from build123d import *

# Parameters (mm, degrees)
F1_DEPTH = 12.7
F2_R     = 2.032
F3_DEPTH = 101.601
F4_R     = 2.032
F5_DEPTH = 101.601
F6_R     = 4.953
F7_DEPTH = 63.246
F9_START = 18.542
F8_R     = 4.953
F9_DEPTH = 49.53


with BuildPart() as f1:
    # F0 (on Top) → F1 (new body)
    with BuildSketch(Plane.XY):
        with BuildLine():
            Line((101.6, 99.2), (101.6, 101.6))
            Line((101.6, 101.6), (0, 101.6))
            Line((0, 101.6), (0, 0))
            Line((0, 0), (2.4, 0))
            ThreePointArc((2.4, 0), (31.4550073063, 70.1449926937), (101.6, 99.2))
        make_face()
        with BuildLine():
            Line((2.4, 99.2), (79.6473236256, 99.2))
            ThreePointArc((79.6473236256, 99.2), (29.7579510314, 71.8420489686), (2.4, 21.9526763744))
            Line((2.4, 21.9526763744), (2.4, 99.2))
        make_face(mode=Mode.SUBTRACT)
    extrude(amount=F1_DEPTH)

    # F2 (on Right) → F3 (cut, through all)
    with BuildSketch(Plane.YZ):
        with Locations((19.05, 6.35)):
            Circle(F2_R)
        with BuildLine():
            ThreePointArc((88.532, 6.35), (86.5, 8.382), (84.468, 6.35))
            ThreePointArc((84.468, 6.35), (86.5, 4.318), (88.532, 6.35))
        make_face()
    extrude(amount=F3_DEPTH, mode=Mode.SUBTRACT)

    # F4 (on Front) → F5 (cut, through all)
    with BuildSketch(Plane.XZ):
        with Locations((15.1, 6.35)):
            Circle(F4_R)
        with Locations((88.9, 6.35)):
            Circle(F4_R)
    extrude(amount=-F5_DEPTH, mode=Mode.SUBTRACT)

    # F6 (on Front) → F7 (cut)
    with BuildSketch(Plane.XZ):
        with Locations((15.1, 6.35)):
            Circle(F6_R)
    extrude(amount=-F7_DEPTH, mode=Mode.SUBTRACT)

    # F8 (on Right) → F9 (cut)
    with BuildSketch(Plane.YZ.offset(F9_START)):
        with Locations((86.5, 6.35)):
            Circle(F8_R)
    extrude(amount=F9_DEPTH, mode=Mode.SUBTRACT)


solid = f1.part
Read the model definition and answer for the solid it produces. Units are mm, in the model's axes. A direction names the side the tool comes from. Round coordinates to 2 decimals unless told otherwise and drop trailing zeros. Order: outer loops, then holes, each group sorted by start corner. A loop starts at its lowest first (then second) coordinate and runs counter-clockwise, first axis right, second up.
1) Flat-ended cylindrical pins translate along their axes: pin 1 (6 mm diameter, centred on y = 42.5, z = 9, fed in from +X); pin 2 (5.5 mm diameter, centred on y = 19.05, z = 6.35, fed in from +X) (3 decimals); pin 3 (1 mm diameter, centred on y = 86.5, z = 3, fed in from +X). Find the tip coordinate at first contact, or state that the pin passes through.
2) The part is cut by section D-D on z = 6.35. Give the number of separate pieces and of enclosed holes in the cut face, plus the area to 3 significant figures.
3) The part is cut by section C-C on y = 86.5. Write down the section's boundary in (x, z).
4) Straight lines are drawn through the part: L1, parallel to Y at x = 1.25, z = 6.35; L2, parallel to Z at x = 3.55, y = 19.05; L3, parallel to Y at x = 17, z = 10.25. For each, find the intervals that lie inside material, in ascending order.
5) For faces 4 (the face through (30.69, 69.37, 6.26)), 5 (the face through (13.07, 49.47, 1.83)), 6 (the face through (52.852, 88.913, 2.025)), 7 (the face through (2.4, 60, 6)), determine the directions among +Z, -Z, +X, -X, +Y, -Y from which every point of the face is accessible in a straight line to the end or side of a thin tool.
6) The part is cut by section A-A on y = 28. Write down the section's boundary in (x, z), plus the area to 3 significant figures.
7) The mould has two halves that part along Z. Classify faces 1 (the face through (39.3, 77.4, 12.7)), 2 (the face through (2.3, 20.927, 5.572)), 3 (the face through (1, 0, 6)): released by +Z, released by -Z, zero draft, split by the parting line, or undercut.
8) The part is cut by section B-B on x = 15.1. Write down the section's boundary in (y, z), plus the area to 3 significant figures.
Resolved:
1. pin 1: stops at x = 13.11
1. pin 2: stops at x = 4.825
1. pin 3: stops at x = 2.4
2. separate pieces: 6
2. enclosed holes: 0
2. area: 645 mm2
3. outline: (0, 0) - (2.4, 0) - (2.4, 4.32) - (0, 4.32) - close; (0, 8.38) - (2.4, 8.38) - (2.4, 12.7) - (0, 12.7) - close; (48.31, 0) - (53.04, 0) - (53.04, 1.4) - (48.31, 1.4) - close; (48.31, 11.3) - (53.04, 11.3) - (53.04, 12.7) - (48.31, 12.7) - close
4. L1: y = 0 to 17.02, 21.08 to 84.47, 88.53 to 101.6
4. L2: z = 0 to 4.32, 8.38 to 12.7
4. L3: y = 99.2 to 101.6
5. face 4: +Z, -Z, +X, -Y
5. face 5: -Y
5. face 6: +X
5. face 7: +Z, -Z
6. outline: (0, 0) - (2.4, 0) - (2.4, 12.7) - (0, 12.7) - close; (3.93, 0) - (6.43, 0) - (6.43, 12.7) - (3.93, 12.7) - close
6. area: 62.2 mm2
7. face 1: released by +Z
7. face 2: undercut
7. face 3: zero draft
8. outline: (48.56, 0) - (53.29, 0) - (53.29, 1.4) - (48.56, 1.4) - close; (48.56, 11.3) - (53.29, 11.3) - (53.29, 12.7) - (48.56, 12.7) - close; (99.2, 0) - (101.6, 0) - (101.6, 4.32) - (99.2, 4.32) - close; (99.2, 8.38) - (101.6, 8.38) - (101.6, 12.7) - (99.2, 12.7) - close
8. area: 33.9 mm2
